Read the model definition and answer for the solid it produces. Units are mm, in the model's axes. A direction names the side the tool comes from. Give positions to 0.01 mm unless a question says otherwise; leave off trailing zeros. Write each loop counter-clockwise with the first axis right and the second up, starting at its lowest first coordinate (ties: lowest second). Pieces come first, ordered by that corner, then holes. Notation, with made-up numbers: (-6.5, 41.5) -> (19.5, 41.5) arc R17 ccw to (19.5, 50.5) -> close; hole circle Ø8 at (75, -21). An arc over 180 degrees is marked (long way). Use a Markdown table: item, result.
from build123d import *

# Parameters (mm, degrees)
BASE_EXTRUDE_DEPTH = 12.7
SKETCH2_R          = 4.7625
CUT_EXTRUDE1_DEPTH = 135.554087638
SKETCH3_R          = 4.7625
CUT_EXTRUDE2_DEPTH = 135.554087638
CHAMFER1_SIZE      = 11.43
CHAMFER1_SIZE2     = 42.657340731
SKETCH4_W          = 101.6
SKETCH4_H          = 25.4
CUT_EXTRUDE3_DEPTH = 3.175
FILLET1_R          = 9.525
FILLET2_R          = 6.35
CHAMFER2_SIZE      = 3.175
SKETCH5_R          = 9.525
CUT_EXTRUDE4_DEPTH = 4.445


with BuildPart() as part:
    # Sketch1 → Base-Extrude (new body)
    with BuildSketch(Plane.XY):
        Polygon((-114.3, 12.7), (12.7, 12.7), (12.7, -69.85), (-25.4, -69.85), (-25.4, -57.15), (-12.7, -57.15), (-12.7, -12.7), (-114.3, -12.7), align=None)
    extrude(amount=BASE_EXTRUDE_DEPTH)

    # Sketch2 → Cut-Extrude1 (cut, through all)
    with BuildSketch(Plane.XY.offset(12.7)):
        Circle(SKETCH2_R)
    extrude(amount=-CUT_EXTRUDE1_DEPTH, mode=Mode.SUBTRACT)

    # Sketch3 → Cut-Extrude2 (cut, through all)
    with BuildSketch(Plane.XY.offset(12.7)):
        with Locations((-106.68, 3.175)):
            Circle(SKETCH3_R)
    extrude(amount=-CUT_EXTRUDE2_DEPTH, mode=Mode.SUBTRACT)

    # Chamfer1
    chamfer1_edges = [part.edges().sort_by_distance(p)[0] for p in [
        (-114.3, -12.7, 6.35),
    ]]
    chamfer1_side = [part.faces().sort_by_distance(p)[0] for p in [
        (-114.3, 0, 6.35),
    ]]
    chamfer(chamfer1_edges, length=CHAMFER1_SIZE, length2=CHAMFER1_SIZE2, reference=chamfer1_side[0])

    # Sketch4 → Cut-Extrude3 (cut)
    with BuildSketch(Plane.XY.offset(12.7)):
        with Locations((-63.5, 0)):
            Rectangle(SKETCH4_W, SKETCH4_H)
    extrude(amount=-CUT_EXTRUDE3_DEPTH, mode=Mode.SUBTRACT)

    # Fillet1
    fillet1_edges = [part.edges().sort_by_distance(p)[0] for p in [
        (12.7, -69.85, 6.35),
    ]]
    fillet(fillet1_edges, radius=FILLET1_R)

    # Fillet2
    fillet2_edges = [part.edges().sort_by_distance(p)[0] for p in [
        (-12.7, -12.7, 4.7625),
    ]]
    fillet(fillet2_edges, radius=FILLET2_R)

    # Chamfer2
    chamfer2_edges = [part.edges().sort_by_distance(p)[0] for p in [
        (12.7, -23.8125, 0),
        (9.910192091, -67.060192091, 0),
        (-50.8, 12.7, 0),
        (-11.1125, -69.85, 0),
    ]]
    chamfer(chamfer2_edges, length=CHAMFER2_SIZE)

    # Sketch5 → Cut-Extrude4 (cut)
    with BuildSketch(Plane(origin=(0, 0, 0), x_dir=(-1, 0, 0), z_dir=(0, 0, -1))):
        Circle(SKETCH5_R)
    extrude(amount=-CUT_EXTRUDE4_DEPTH, mode=Mode.SUBTRACT)


solid = part.part
Item 1: A tool of negligible diameter and unlimited length cuts with its end or side. For faces 4 (the face through (-12.7, -30, 8)), 5 (the face through (-25.4, -64, 6)), 6 (the face through (-19, -57.15, 6)), 7 (the face through (7.559, -5.796, 2.191)), from which of +Z, -Z, +X, -X, +Y, -Y can it reach the whole face along a straight path? Write none if from no direction.
Return value:
| item | result |
|---|---|
| face 4 | +Z, -X |
| face 5 | +Z, -Z, -X, -Y |
| face 6 | +Z, -Z, -X |
| face 7 | -Z |
Item 2: A cutting plane is placed at C-C (x = -28). Give the vertices of the cut face in (y, z) (3 decimals).
Return value:
| item | result |
|---|---|
| outline | (-12.7, 0) -> (9.525, 0) -> (12.7, 3.175) -> (12.7, 9.525) -> (-12.7, 9.525) -> close |
Item 3: For a pull along Y with two mould halves and no side action, classify faces 1 (the face through (-38, -11, 0)), 2 (the face through (8.58, -65.61, 1.21)), 3 (the face through (-3.78, -2.9, 8.63)) as +Y half, -Y half, draft (parallel to the pull), parting line (faces both ways), or undercut.
Return value:
| item | result |
|---|---|
| face 1 | draft |
| face 2 | -Y half |
| face 3 | undercut |
Item 4: Straight lines are drawn through the part: line 1 along Y through (x, z) = (0, 10); line 2 along X through (y, z) = (0, 1.1) (3 decimals); line 3 along Z through (x, y) = (-35.5, 6.5) (3 decimals). For each, find the intervals that lie inside material, in ascending order. Write a range as [from, to].
Return value:
| item | result |
|---|---|
| line 1 | [-69.85, -4.76], [4.76, 12.7] |
| line 2 | [-114.3, -110.23], [-103.13, -9.525], [9.525, 10.625] |
| line 3 | [0, 9.525] |
Item 5: A cutting plane is placed at B-B (x = -106.68). Give the vertices of the cut face in (y, z) (1 decimal).
Return value:
| item | result |
|---|---|
| outline | (-3.3, 0) -> (-1.6, 0) -> (-1.6, 9.5) -> (-3.3, 9.5) -> close; (7.9, 0) -> (9.5, 0) -> (12.7, 3.2) -> (12.7, 9.5) -> (7.9, 9.5) -> close |
Item 6: Each of these flat-tipped pins is pushed along its axis until it touches: P1, Ø9.5, axis at x = 4.5, y = 1.5, coming from the -Z side (3 decimals); P2, Ø2, axis at x = -53.5, z = 1.5, coming from the +Y side (3 decimals); P3, Ø7.5, axis at x = -106.68, y = 3.175, coming from the +Z side; P4, Ø6, axis at x = -55.5, z = 10.5, coming from the -Y side. Where does it stop, or does it pass through?
Return value:
| item | result |
|---|---|
| P1 | z = 4.445 |
| P2 | y = 12.025 |
| P3 | through |
| P4 | y = -12.7 |
Item 7: A cutting plane is placed at A-A (y = -41). Give the vertices of the cut face in (x, z) (3 decimals).
Return value:
| item | result |
|---|---|
| outline | (-12.7, 0) -> (9.525, 0) -> (12.7, 3.175) -> (12.7, 12.7) -> (-12.7, 12.7) -> close |
